Model file for the job. Use its own axes, mm. Face numbers are marked on the shaded views. Give positions to 0.01 mm unless a question says otherwise; leave off trailing zeros. Loops run counter-clockwise (first coordinate to the right, second up) from the corner with the lowest first, then second, coordinate; pieces in that order, holes last. Notation, with made-up numbers: M 64.25,-28.75 L 120.25,-28.75 A16 cw 120.25,-24.75 Z; hole C 50.5,-22.5 d2. An arc over 180 degrees is marked long. Answer in a Markdown table with one row per item.
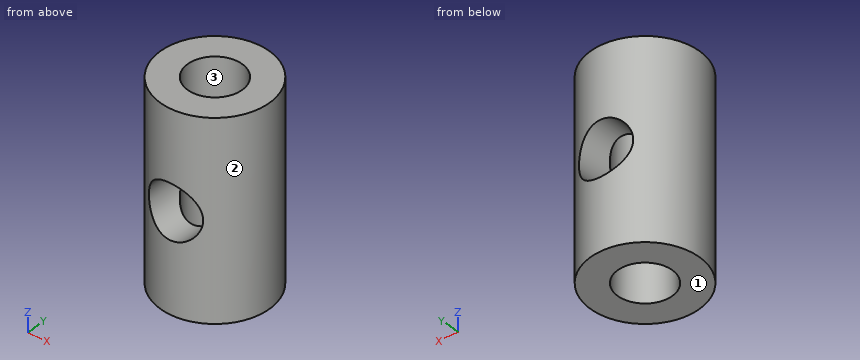
```python
from build123d import *

# Parameters (mm, degrees)
SKETCH1_R               = 50
SKETCH1_R_2             = 25
BOSS_EXTRUDE1_DEPTH     = 90
CUT_EXTRUDE1_DEPTH      = 115.455231423
CUT_EXTRUDE1_DEPTH_BACK = 115.455231423
SKETCH2_R               = 25


with BuildPart() as part:
    # Sketch1 → Boss-Extrude1 (new, symmetric)
    with BuildSketch(Plane.XY):
        with Locations(Location((0, 0, 0), (0, 0, 180))):
            Circle(SKETCH1_R)
        with Locations(Location((0, 0, 0), (0, 0, 180))):
            Circle(SKETCH1_R_2, mode=Mode.SUBTRACT)
    extrude(amount=BOSS_EXTRUDE1_DEPTH, both=True)

    # Sketch2 → Cut-Extrude1 (cut, two sides: drawn at the far end of the back side and taken through both)
    with BuildSketch(Plane(origin=(0, 0, 0), x_dir=(1, 0, 0), z_dir=(0, 1, 0)).offset(-CUT_EXTRUDE1_DEPTH_BACK)):
        with Locations(Location((0, 0, 0), (0, 0, 270))):
            Circle(SKETCH2_R)
    extrude(amount=CUT_EXTRUDE1_DEPTH + CUT_EXTRUDE1_DEPTH_BACK, mode=Mode.SUBTRACT)


solid = part.part
```
(1) Saw through at B-B, the plane z = -21. Give the cut face in (x, y), and give its area (3 significant figures).
Established:
| item | result |
|---|---|
| outline | M -13.56,-48.12 L -13.56,-21 A25 cw -13.56,21 L -13.56,48.12 A50 ccw Z; M 13.56,-48.12 A50 ccw 13.56,48.12 L 13.56,21 A25 cw 13.56,-21 Z |
| area | 4,500 mm2 |
(2) Saw through at D-D, the plane y = 39. Give the cut face in (x, z), and give its area (3 significant figures).
Established:
| item | result |
|---|---|
| outline | M -31.29,-90 L 31.29,-90 L 31.29,90 L -31.29,90 Z; hole C 0,0 d50 |
| area | 9,300 mm2 |
(3) Wall check: L1, parallel to Y at x = 0, z = 34.5; L2, parallel to Z at x = 0, y = 37; L3, parallel to Y at x = -4, z = 69.5. Give the ranges that are in metal, low to high.
Established:
| item | result |
|---|---|
| L1 | y = -50 to -25, 25 to 50 |
| L2 | z = -90 to -25, 25 to 90 |
| L3 | y = -49.84 to -24.68, 24.68 to 49.84 |
(4) Saw through at C-C, the plane y = 5. Give the cut face in (x, z).
Established:
| item | result |
|---|---|
| outline | M -49.75,-90 L -24.49,-90 L -24.49,-5 A25 cw -24.49,5 L -24.49,90 L -49.75,90 Z; M 24.49,-90 L 49.75,-90 L 49.75,90 L 24.49,90 L 24.49,5 A25 cw 24.49,-5 Z |
(5) Mould opens along Y. For the marked faces 1, 2 and 3 say: pulls with the +Y half, pulls with the -Y half, needs draft (parallel to the pull), parting line crosses it, or undercut.
Established:
| item | result |
|---|---|
| face 1 | needs draft |
| face 2 | parting line crosses it |
| face 3 | undercut |
(6) Flat gauge pins, fed straight in: P1, Ø4, axis at y = 32, z = -54.5, coming from the -X side; P2, Ø12, axis at y = -16, z = -1.5, coming from the +X side; P3, Ø3, axis at x = 15.5, z = 72, coming from the +Y side. Where does each tip first touch, or does it go through?
Established:
| item | result |
|---|---|
| P1 | stops at x = -40 |
| P2 | stops at x = 48.99 |
| P3 | stops at y = 48 |
(7) Saw through at A-A, the plane x = 0. Give the cut face in (y, z).
Established:
| item | result |
|---|---|
| outline | M -50,-90 L -25,-90 L -25,-25 L -50,-25 Z; M -50,25 L -25,25 L -25,90 L -50,90 Z; M 25,-90 L 50,-90 L 50,-25 L 25,-25 Z; M 25,25 L 50,25 L 50,90 L 25,90 Z |
